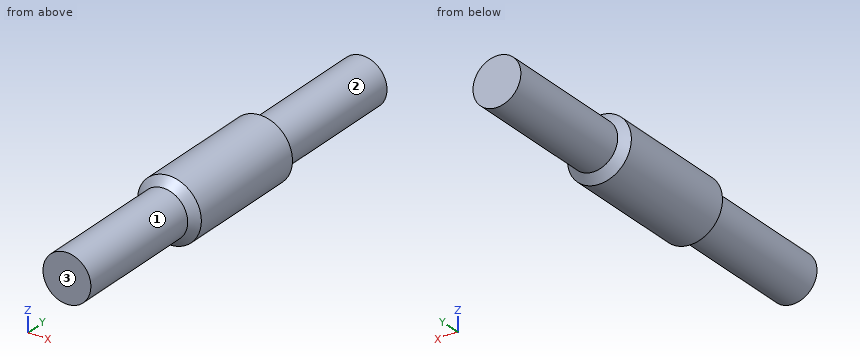
from build123d import *

# Parameters (mm, degrees)
SKETCH_1_R      = 2
EXTRUDE_1_DEPTH = 10
SKETCH_2_R      = 1.5
EXTRUDE_2_DEPTH = 8
EXTRUDE_START   = 8
SKETCH_3_R      = 1.5
EXTRUDE_3_DEPTH = 8
CHAMFER_1_SIZE  = 1


with BuildPart() as part:
    # 草图1 → 凸台-拉伸1 (new body)
    with BuildSketch(Plane(origin=(0, 0, 0), x_dir=(1, 0, 0), z_dir=(0, 1, 0))):
        with Locations(Location((0, 0, 0), (0, 0, 270))):
            Circle(SKETCH_1_R)
    extrude(amount=EXTRUDE_1_DEPTH)

    # 草图2 → 凸台-拉伸2 (add)
    with BuildSketch(Plane.XZ):
        with Locations(Location((0, 0, 0), (0, 0, 270))):
            Circle(SKETCH_2_R)
    extrude(amount=EXTRUDE_2_DEPTH)

    # 草图3 → 凸台-拉伸3 (add)
    with BuildSketch(Plane(origin=(0, 10, 0), x_dir=(1, 0, 0), z_dir=(0, 1, 0)).offset(EXTRUDE_START)):
        with Locations(Location((0, 0, 0), (0, 0, 90))):
            Circle(SKETCH_3_R)
    extrude(amount=-EXTRUDE_3_DEPTH)

    # 倒角1
    # the kernel refuses this chamfer: 1 mm, written as the material it takes off along each edge
    with BuildSketch(Plane(origin=(0, 0, 0), x_dir=(0, 0, 1), z_dir=(-1, 0, 0))) as chamfer_1_piece_1_section:
        Polygon((2, CHAMFER_1_SIZE), (2 - CHAMFER_1_SIZE, 0), (2, 0), align=None)
    chamfer_1_piece_1 = revolve(axis=Axis((0, 0, 0), (0, 1, 0)), mode=Mode.PRIVATE)
    chamfer_1_piece_1 = chamfer_1_piece_1 - Plane(origin=(0, 0.752378324, 0), x_dir=(0, 0, -1), z_dir=(0, 1, 0)) * Cylinder(1.5, 8, mode=Mode.PRIVATE)
    add(chamfer_1_piece_1, mode=Mode.SUBTRACT)
    with BuildSketch(Plane(origin=(0, 10, 0), x_dir=(0, 0, 1), z_dir=(-1, 0, 0))) as chamfer_1_piece_2_section:
        Polygon((2, -CHAMFER_1_SIZE), (2 - CHAMFER_1_SIZE, 0), (2, 0), align=None)
    chamfer_1_piece_2 = revolve(axis=Axis((0, 10, 0), (0, 1, 0)), mode=Mode.PRIVATE)
    chamfer_1_piece_2 = chamfer_1_piece_2 - Plane(origin=(0, 9.247621676, 0), x_dir=(0, 0, -1), z_dir=(0, 1, 0)) * Cylinder(1.5, 8, mode=Mode.PRIVATE)
    add(chamfer_1_piece_2, mode=Mode.SUBTRACT)


solid = part.part
Geometry check sheet. Reference: the model listing, model coordinates, mm. Face numbers are marked on the shaded views. A direction names the side the tool comes from. Give positions to 0.01 mm unless a question says otherwise; leave off trailing zeros. Loops run counter-clockwise (first coordinate to the right, second up) from the corner with the lowest first, then second, coordinate; pieces in that order, holes last. Notation, with made-up numbers: (80.5, 16) -> (114.5, 16) arc R28 ccw to (114.5, 42) -> close; hole circle Ø2 at (69.25, -36). An arc over 180 degrees is marked (long way). Answer in a Markdown table with one row per item. Add a question column.
1) Gauge pin test, flat ends, axial feed: P1, Ø2, axis at x = -1, y = 13.5, coming from the +Z side; P2, Ø1, axis at x = -1.5, y = -4, coming from the -Z side. Record the tip position at first contact, or that the pin passes through.
2) Cross-section at A-A on z = 0. Record the boundary of the cut face in (x, y), and give its area (3 significant figures).
3) Set-up check for the marked faces 1, 2 and 3: record each of +Z, -Z, +X, -X, +Y, -Y from which the full face is reachable in a straight line by a thin tool's end or side.
4) Cross-section at B-B on x = 0. Record the boundary of the cut face in (y, z).
5) Material ranges on probe 1 along X at (y, z) = (-3.25, -0.45); probe 2 along Y at (x, z) = (-1.65, -0.2); probe 3 along X at (y, z) = (-3.75, -0.3), recorded low to high. Write a range as from..to.
6) Cross-section at C-C on y = -5. Record the boundary of the cut face in (x, z), and give its area (3 significant figures).
Outcome:
| question | item | result |
|---|---|---|
| 1 | P1 | stops at z = 1.5 |
| 1 | P2 | stops at z = -1.12 |
| 2 | outline | (-2, 1) -> (-1.5, 0.5) -> (-1.5, -8) -> (1.5, -8) -> (1.5, 0.5) -> (2, 1) -> (2, 9) -> (1.5, 9.5) -> (1.5, 18) -> (-1.5, 18) -> (-1.5, 9.5) -> (-2, 9) -> close |
| 2 | area | 86.5 mm^2 |
| 3 | face 1 | -Y |
| 3 | face 2 | +Y |
| 3 | face 3 | +Z, -Z, +X, -X, -Y |
| 4 | outline | (-8, -1.5) -> (0.5, -1.5) -> (1, -2) -> (9, -2) -> (9.5, -1.5) -> (18, -1.5) -> (18, 1.5) -> (9.5, 1.5) -> (9, 2) -> (1, 2) -> (0.5, 1.5) -> (-8, 1.5) -> close |
| 5 | probe 1 | x = -1.43..1.43 |
| 5 | probe 2 | y = 0.66..9.34 |
| 5 | probe 3 | x = -1.47..1.47 |
| 6 | outline | circle Ø3 at (0, 0) |
| 6 | area | 7.07 mm^2 |
